Check sheet for the drawn part. Datum: minimum x, y, z corner. Units: mm. A direction names the side the tool comes from. Give positions to 0.01 mm unless a question says otherwise; leave off trailing zeros. Write each loop counter-clockwise with the first axis right and the second up, starting at its lowest first coordinate (ties: lowest second). Pieces come first, ordered by that corner, then holes.
(1) Cross-section at D-D (z = 46). Record the boundary of the cut face in (x, y), and give its area (3 significant figures).
(2) Tool access check on the marked faces 1, 2 and 3. Record the directions out of +Z, -Z, +X, -X, +Y, -Y that give a thin tool (end or side, any length) a straight path to the whole face; none if there is none.
(3) Cross-section at A-A (z = 26). Record the boundary of the cut face in (x, y).
(4) Thickness scan on line 1 along Z through (x, y) = (75, 76); line 2 along Y through (x, z) = (17, 33); line 3 along X through (y, z) = (5, 33). Record the ranges inside material, lowest first.
(5) Cross-section at C-C (y = 34.5). Record the boundary of the cut face in (x, z), and give its area (3 significant figures).
(6) Depth check by flat-ended pin: P1, Ø8, axis at x = 87, y = 28, coming from the +Z side; P2, Ø5, axis at y = 3.5, z = 33.5, coming from the +X side; P3, Ø24, axis at x = 16.5, z = 35.5, coming from the +Y side. Enter the tip coordinate at first touch or a pass-through.
(7) Cross-section at B-B (x = 112.5). Record the boundary of the cut face in (y, z), and give its area (3 significant figures).
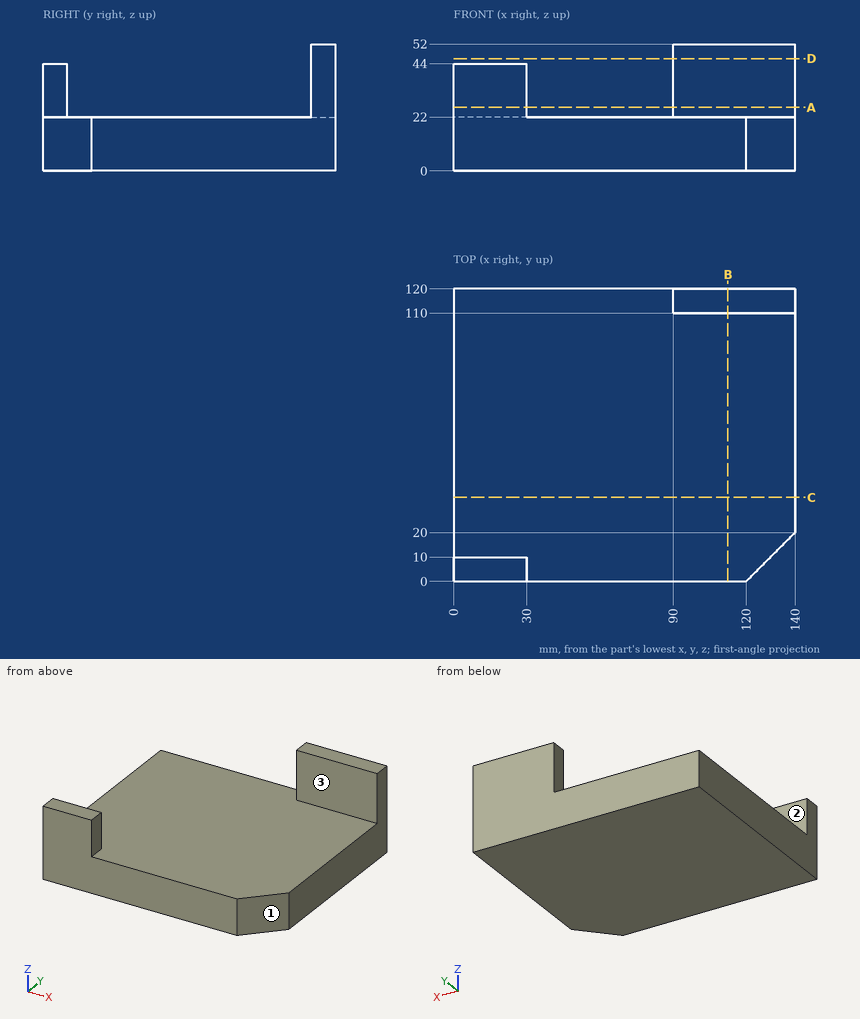
Reply:
1. outline: (90, 110) - (140, 110) - (140, 120) - (90, 120) - close
1. area: 500 mm2
2. face 1: +Z, -Z, +X, -Y
2. face 2: +Z, +X, -X, +Y
2. face 3: +Z, +X, -X, -Y
3. outline: (0, 0) - (30, 0) - (30, 10) - (0, 10) - close; (90, 110) - (140, 110) - (140, 120) - (90, 120) - close
4. line 1: z = 0 to 22
4. line 2: y = 0 to 10
4. line 3: x = 0 to 30
5. outline: (0, 0) - (140, 0) - (140, 22) - (0, 22) - close
5. area: 3,080 mm2
6. P1: stops at z = 22
6. P2: stops at x = 30
6. P3: stops at y = 10
7. outline: (0, 0) - (120, 0) - (120, 52) - (110, 52) - (110, 22) - (0, 22) - close
7. area: 2,940 mm2
